The model under review builds one solid part; all positions refer to its coordinate system, in mm. A direction names the side the tool comes from. Coordinates: 2 decimals unless noted, no trailing zeros. Loops run counter-clockwise (first coordinate to the right, second up) from the corner with the lowest first, then second, coordinate; pieces in that order, holes last. Notation, with made-up numbers: (29, 5.25) - (80, 5.25) arc R31 cw to (80, 31.25) - close; hole circle Ø7 at (48.5, 65.25). An arc over 180 degrees is marked (long way). Answer in a Markdown table with one row per item. Add a question column.
(1) For P1, Ø8, axis at x = -91, y = 117, coming from the +Z side; P2, Ø12, axis at x = 99.5, y = 224.5, coming from the +Z side; P3, Ø8, axis at y = 54, z = 645, coming from the -X side, all flat-tipped, find the tip position at first contact; note any pin that passes through.
(2) Machinability: for faces 4 (the flat face through (2, -133.966, 541)), 5 (the flat face through (2, 74, 0)), which of the approach directions +Z, -Z, +X, -X, +Y, -Y give a long, thin tool a straight path to every point of the face, cutting with its end or side? Answer none if there is none.
(3) We need section B-B on x = 170.5. Write out the cut boundary in (y, z).
(4) We need section C-C on z = 507.5. Write out the cut boundary in (x, y).
(5) For line 1 along X through (y, z) = (93.5, 461.5); line 2 along Y through (x, z) = (237, 619.5); line 3 along Z through (x, y) = (-13, 197), list the stretches that pass through material, from the lowest coordinate up.
(6) We need section D-D on y = 209. Write out the cut boundary in (x, z), plus the area to 3 significant figures.
(7) Mouldability with a two-part tool opening along Y and no side actions: class faces 1 (the cylindrical face through (-0.606, 226.747, 735.642)), 2 (the flat face through (2, 316.034, 316)), 3 (the flat face through (2, 176.034, 541)) as +Y half, -Y half, draft (parallel to the pull), parting line (faces both ways), or undercut.
(8) We need section A-A on y = -108.5. Write out the cut boundary in (x, z).
from build123d import *

# Parameters (mm, degrees)
F0_W     = 600
F0_H     = 490
F1_DEPTH = 640
F2_W     = 520
F2_H     = 310
F3_DEPTH = 200
F4_R     = 30
F5_DEPTH = 194


with BuildPart() as f1:
    # F0 (on Top) → F1 (new body)
    with BuildSketch(Plane.XY):
        with Locations((5.897177, 71.033585)):
            Rectangle(F0_W, F0_H)
    extrude(amount=F1_DEPTH)

    # F2 (on face) → F3 (cut)
    with BuildSketch(Plane.XY.offset(640)):
        with Locations((5.897177, 21.033585)):
            Rectangle(F2_W, F2_H)
    extrude(amount=-F3_DEPTH, mode=Mode.SUBTRACT)

    # F4 (on face) → F5 (join)
    with BuildSketch(Plane.XY.offset(640)):
        with Locations((5.897177, 256.033585)):
            Circle(F4_R)
    extrude(amount=F5_DEPTH)


solid = f1.part
Outcome:
| question | item | result |
|---|---|---|
| 1 | P1 | z = 440 |
| 1 | P2 | z = 640 |
| 1 | P3 | through |
| 2 | face 4 | +Z |
| 2 | face 5 | -Z, +X, -X, +Y, -Y |
| 3 | outline | (-173.97, 0) - (316.03, 0) - (316.03, 640) - (176.03, 640) - (176.03, 440) - (-133.97, 440) - (-133.97, 640) - (-173.97, 640) - close |
| 4 | outline | (-294.1, -173.97) - (305.9, -173.97) - (305.9, 316.03) - (-294.1, 316.03) - close; hole (-254.1, -133.97) - (265.9, -133.97) - (265.9, 176.03) - (-254.1, 176.03) - close |
| 5 | line 1 | -294.1 to -254.1, 265.9 to 305.9 |
| 5 | line 2 | -173.97 to -133.97, 176.03 to 316.03 |
| 5 | line 3 | 0 to 640 |
| 6 | outline | (-294.1, 0) - (305.9, 0) - (305.9, 640) - (-294.1, 640) - close |
| 6 | area | 384,000 mm² |
| 7 | face 1 | parting line |
| 7 | face 2 | +Y half |
| 7 | face 3 | undercut |
| 8 | outline | (-294.1, 0) - (305.9, 0) - (305.9, 640) - (265.9, 640) - (265.9, 440) - (-254.1, 440) - (-254.1, 640) - (-294.1, 640) - close |
